Read the model definition and answer for the solid it produces. Units are mm, in the model's axes. A direction names the side the tool comes from. Give positions to 0.01 mm unless a question says otherwise; leave off trailing zeros. Write each loop counter-clockwise with the first axis right and the second up, starting at its lowest first coordinate (ties: lowest second). Pieces come first, ordered by that corner, then holes. Notation, with made-up numbers: (-2.5, 31.5) - (44.5, 31.5) arc R20 ccw to (44.5, 65.5) - close; hole circle Ø7 at (89, -20.75). An arc over 180 degrees is marked (long way). Answer as CSV lines item,"result".
```python
from build123d import *

# Parameters (mm, degrees)
F1_DEPTH = 2
F2_DEPTH = 2
F3_DEPTH = 10


with BuildPart() as f1:
    # F0 (on Top) → F1 (new body)
    with BuildSketch(Plane.XY):
        with BuildLine():
            Line((0, 2), (0, 7))
            ThreePointArc((0, 7), (-7, 0), (0, -7))
            Line((0, -7), (0, -2))
            ThreePointArc((0, -2), (-2, 0), (0, 2))
        make_face()
    extrude(amount=F1_DEPTH)



with BuildPart() as f2:
    # F0 (on Top) → F2 (new body)
    with BuildSketch(Plane.XY):
        with BuildLine():
            ThreePointArc((0, -7), (4.949747, -4.949747), (7, 0))
            ThreePointArc((7, 0), (4.949747, 4.949747), (0, 7))
            Line((0, 7), (0, 2))
            ThreePointArc((0, 2), (1.414214, 1.414214), (2, 0))
            ThreePointArc((2, 0), (1.414214, -1.414214), (0, -2))
            Line((0, -2), (0, -7))
        make_face()
    extrude(amount=F2_DEPTH)


with BuildPart() as f1_1:
    add(f1.part)

    add(f2.part)  # F3 merges F2
    # F0 (on Top) → F3 (join)
    with BuildSketch(Plane.XY):
        with BuildLine():
            ThreePointArc((2, 0), (1.414214, 1.414214), (0, 2))
            Line((0, 2), (0, 1))
            ThreePointArc((0, 1), (0.707107, 0.707107), (1, 0))
            ThreePointArc((1, 0), (0.707107, -0.707107), (0, -1))
            Line((0, -1), (0, -2))
            ThreePointArc((0, -2), (1.414214, -1.414214), (2, 0))
        make_face()
        with BuildLine():
            Line((0, 1), (0, 2))
            ThreePointArc((0, 2), (-2, 0), (0, -2))
            Line((0, -2), (0, -1))
            ThreePointArc((0, -1), (-1, 0), (0, 1))
        make_face()
    extrude(amount=F3_DEPTH)


solid = f1_1.part
```
(1) Find the intervals of material crossed by L1, parallel to Z at x = -4.5, y = 3.25; L2, parallel to Y at x = 0.5, z = 7.5; L3, parallel to Y at x = -0.75, z = 7.5, in increasing order.
Worked out:
L1,"z = 0 to 2"
L2,"y = -1.94 to -0.87, 0.87 to 1.94"
L3,"y = -1.85 to -0.66, 0.66 to 1.85"
(2) A cutting plane is placed at A-A (z = 8.5). Write down the section's boundary in (x, y), and give its area (3 significant figures).
Worked out:
outline,"(0, -2) arc R2 ccw to (2, 0) arc R2 ccw to (0, 2) arc R2 ccw to start; hole (0, 1) arc R1 ccw (long way) to (1, 0) arc R1 ccw to start"
area,"9.42 mm^2"
(3) A cutting plane is placed at D-D (y = -5.75). Write down the section's boundary in (x, z), and give its area (3 significant figures).
Worked out:
outline,"(-3.99, 0) - (3.99, 0) - (3.99, 2) - (-3.99, 2) - close"
area,"16.0 mm^2"
(4) This flat-tipped pin is pushed along its axis until it touches: P1, Ø1, axis at x = -5.5, y = -2, coming from the +Z side. Where does it stop, or does it pass through?
Worked out:
P1,"stops at z = 2"
(5) A cutting plane is placed at C-C (y = 6). Write down the section's boundary in (x, z), and give its area (3 significant figures).
Worked out:
outline,"(-3.61, 0) - (3.61, 0) - (3.61, 2) - (-3.61, 2) - close"
area,"14.4 mm^2"
(6) For faces 1 (the flat face through (1, -1, 10)), 2 (the flat face through (-2, -1, 2)), determine the directions among +Z, -Z, +X, -X, +Y, -Y from which every point of the face is accessible in a straight line to the end or side of a thin tool.
Worked out:
face 1,"+Z, +X, -X, +Y, -Y"
face 2,"+Z"
(7) A cutting plane is placed at B-B (y = 0.25). Write down the section's boundary in (x, z).
Worked out:
outline,"(-7, 0) - (-0.97, 0) - (-0.97, 10) - (-1.98, 10) - (-1.98, 2) - (-7, 2) - close; (0.97, 0) - (7, 0) - (7, 2) - (1.98, 2) - (1.98, 10) - (0.97, 10) - close"
